Geometry: final body of the model. Coordinates: model frame, mm. Face numbers are marked on the shaded views. A direction names the side the tool comes from. Coordinates: 2 decimals unless noted, no trailing zeros. Loops run counter-clockwise (first coordinate to the right, second up) from the corner with the lowest first, then second, coordinate; pieces in that order, holes last. Notation, with made-up numbers: (-8, -2.5) - (27, -2.5) arc R15 ccw to (27, 5.5) - close; hole circle Ø9 at (-16, 48.25). An arc over 180 degrees is marked (long way). Put each result on its own line as item: value. Start each with the question number.
1) Section D-D on y = -56. Output: boundary loops of the cut face in (x, z), and give its area (3 significant figures).
2) Material intervals for line 1 along X through (y, z) = (-26, 27.5); line 2 along Z through (x, y) = (-23.5, -33.5); line 3 along Z through (x, y) = (-4, 0), sorted ascending. Write a range as from..to.
3) Section B-B on z = 30. Output: boundary loops of the cut face in (x, y), and give its area (3 significant figures).
4) Reachability of the marked faces 1, 2, 3, 4 and 5 from +Z, -Z, +X, -X, +Y, -Y: full face, straight path, thin tool, end or side. Return the list, or none.
5) Contact query for flat-ended pins moving along their axis: pin 1 Ø18.5 at (y, z) = (-39.5, 23) entering from +X; pin 2 Ø18.5 at (y, z) = (-23, 20.5) entering from -X; pin 3 Ø14.5 at (x, y) = (32, -2.5) entering from +Z. Output: stop coordinate, or through.
6) Section C-C on x = -13.5. Output: boundary loops of the cut face in (y, z), and give its area (3 significant figures).
7) Section A-A on y = 0. Output: boundary loops of the cut face in (x, z), and give its area (3 significant figures).
```python
from build123d import *

# Parameters (mm, degrees)
F0_W      = 76
F0_H      = 13
F1_DEPTH  = 2
F2_R      = 8
F3_W      = 43
F3_H      = 13
F4_DEPTH  = 9
F5_W      = 43
F5_H      = 36
F6_DEPTH  = 70
F8_DEPTH  = 41
F10_DEPTH = 2
F12_DEPTH = 3
F13_R     = 1.5
F14_DEPTH = 25
F15_W     = 5.5
F15_H     = 13
F16_DEPTH = 42
F17_SIZE  = 3.5


with BuildPart() as f1:
    # F0 (on Top) → F1 (new body)
    with BuildSketch(Plane.XY):
        Rectangle(F0_W, F0_H)
    extrude(amount=F1_DEPTH)

    # F2
    f2_edges = [f1.edges().sort_by_distance(p)[0] for p in [
        (-38, 6.5, 1),
        (38, 6.5, 1),
    ]]
    fillet(f2_edges, radius=F2_R)

    # F3 (on face) → F4 (join)
    with BuildSketch(Plane.XY.offset(2)):
        with Locations((-5, 0)):
            Rectangle(F3_W, F3_H)
    extrude(amount=F4_DEPTH)

    # F5 (on face) → F6 (join)
    with BuildSketch(Plane(origin=(0, 6.5, 0), x_dir=(-1, 0, 0), z_dir=(0, 1, 0))):
        with Locations((5, 29)):
            Rectangle(F5_W, F5_H)
    extrude(amount=-F6_DEPTH)

    # F7 (on face) → F8 (cut)
    with BuildSketch(Plane.YZ.offset(16.5)):
        Polygon((-57.5, 15), (-2.5, 15), (-2.5, 6), (2.5, 6), (2.5, 43), (-57.5, 43), align=None)
    extrude(amount=-F8_DEPTH, mode=Mode.SUBTRACT)

    # F9 (on face) → F10 (join)
    with BuildSketch(Plane.YZ.offset(16.5)):
        Polygon((-63.5, 11), (-6.5, 11), (-6.5, 2), (6.5, 2), (6.5, 47), (-63.5, 47), align=None)
    extrude(amount=F10_DEPTH)

    # F11 (on face) → F12 (join)
    with BuildSketch(Plane.XY.offset(2)):
        with BuildLine():
            Line((-38, -6.5), (-26.5, -6.5))
            Line((-26.5, -6.5), (-26.5, 6.5))
            Line((-26.5, 6.5), (-30, 6.5))
            ThreePointArc((-30, 6.5), (-35.656854, 4.156854), (-38, -1.5))
            Line((-38, -1.5), (-38, -6.5))
        make_face()
        with BuildLine():
            ThreePointArc((38, -1.5), (35.656854, 4.156854), (30, 6.5))
            Line((30, 6.5), (18.5, 6.5))
            Line((18.5, 6.5), (18.5, -6.5))
            Line((18.5, -6.5), (38, -6.5))
            Line((38, -6.5), (38, -1.5))
        make_face()
    extrude(amount=F12_DEPTH)

    # F13 (on face) → F14 (cut)
    with BuildSketch(Plane.XY.offset(5)):
        with Locations((-31.5, 0)):
            Circle(F13_R)
        with Locations((31.5, 0)):
            Circle(F13_R)
    extrude(amount=-F14_DEPTH, mode=Mode.SUBTRACT)

    # F15 (on face) → F16 (join)
    with BuildSketch(Plane.XY.offset(5)):
        with Locations((21.25, 0)):
            Rectangle(F15_W, F15_H)
    extrude(amount=F16_DEPTH)

    # F17
    f17_edges = [f1.edges().sort_by_distance(p)[0] for p in [
        (18.5, -63.5, 29),
        (-4, -63.5, 47),
        (-4, -63.5, 11),
        (-26.5, -63.5, 29),
    ]]
    chamfer(f17_edges, length=F17_SIZE)


solid = f1.part
```
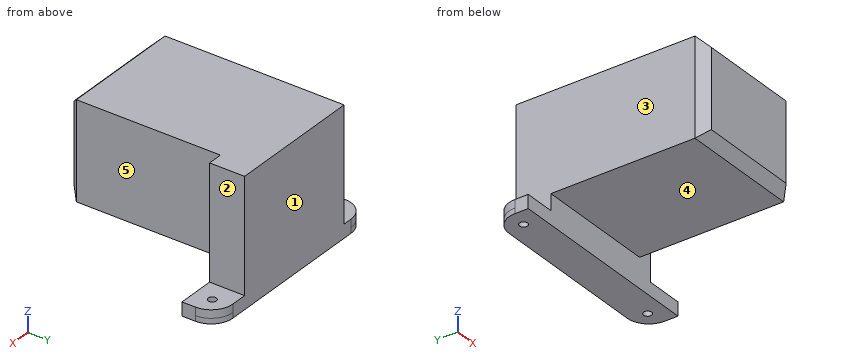
Answer block:
1. outline: (-26.5, 11) - (18.5, 11) - (18.5, 47) - (-26.5, 47) - close; hole (-24.5, 15) - (16.5, 15) - (16.5, 43) - (-24.5, 43) - close
1. area: 472 mm²
2. line 1: x = -26.5..-24.5, 16.5..18.5
2. line 2: z = 11..15, 43..47
2. line 3: z = 0..6, 43..47
3. outline: (-26.5, -60) - (-23, -63.5) - (15, -63.5) - (18.5, -60) - (18.5, -6.5) - (24, -6.5) - (24, 6.5) - (-26.5, 6.5) - close; hole (-24.5, -57.5) - (16.5, -57.5) - (16.5, 2.5) - (-24.5, 2.5) - close
3. area: 749 mm²
4. face 1: +Z, -Z, +X, -X, +Y
4. face 2: +Z, +X, +Y, -Y
4. face 3: +Z, -X, +Y, -Y
4. face 4: -Z, +X, -X, -Y
4. face 5: +Z, -Z, +X, -Y
5. pin 1: stops at x = 18.5
5. pin 2: stops at x = -26.5
5. pin 3: stops at z = 5
6. outline: (-63.5, 14.5) - (-60, 11) - (-6.5, 11) - (-6.5, 0) - (6.5, 0) - (6.5, 47) - (-60, 47) - (-63.5, 43.5) - close; hole (-57.5, 15) - (-2.5, 15) - (-2.5, 6) - (2.5, 6) - (2.5, 43) - (-57.5, 43) - close
6. area: 926 mm²
7. outline: (-37.86, 0) - (-33, 0) - (-33, 5) - (-37.86, 5) - close; (-30, 0) - (30, 0) - (30, 5) - (24, 5) - (24, 47) - (-26.5, 47) - (-26.5, 5) - (-30, 5) - close; (33, 0) - (37.86, 0) - (37.86, 5) - (33, 5) - close; hole (-24.5, 6) - (16.5, 6) - (16.5, 43) - (-24.5, 43) - close
7. area: 953 mm²
